Source: CAD feature listing. Evaluate the final solid. Frame: model axes, mm. A direction names the side the tool comes from. Give positions to 0.01 mm unless a question says otherwise; leave off trailing zeros. Write each loop counter-clockwise with the first axis right and the second up, starting at its lowest first coordinate (ties: lowest second). Pieces come first, ordered by that corner, then holes. Notation, with made-up numbers: (29.5, 30.25) -> (85.5, 30.25) arc R26 ccw to (85.5, 53.25) -> close; hole circle Ø11 at (57, 87.25). An arc over 180 degrees is marked (long way). Write item = value, one per line.
from build123d import *

# Parameters (mm, degrees)
SCHIZZO1_R                   = 3.4
ESTRUSIONE_ESTRUSIONE1_DEPTH = 200


with BuildPart() as part:
    # Schizzo1 → Estrusione-Estrusione1 (new body)
    with BuildSketch(Plane(origin=(0, 0, -1034), x_dir=(-1, 0, 0), z_dir=(0, 0, -1))):
        with BuildLine():
            Line((-16, 3.5), (-16, 1.5))
            ThreePointArc((-16, 1.5), (-15.560660172, 0.439339828), (-14.5, 0))
            Line((-14.5, 0), (-4, 0))
            ThreePointArc((-4, 0), (-1.171572875, 1.171572875), (0, 4))
            Line((0, 4), (0, 14.5))
            ThreePointArc((0, 14.5), (-0.439339828, 15.560660172), (-1.5, 16))
            Line((-1.5, 16), (-3.5, 16))
            ThreePointArc((-3.5, 16), (-4.207106781, 15.707106781), (-4.5, 15))
            Line((-4.5, 15), (-4.5, 13.5))
            ThreePointArc((-4.5, 13.5), (-4.353553391, 13.146446609), (-4, 13))
            Line((-4, 13), (-2.45, 13))
            ThreePointArc((-2.45, 13), (-2.131801948, 12.868198052), (-2, 12.55))
            Line((-2, 12.55), (-2, 12.5))
            ThreePointArc((-2, 12.5), (-2.732233047, 10.732233047), (-4.5, 10))
            Line((-4.5, 10), (-5.807611845, 10))
            ThreePointArc((-5.807611845, 10), (-7.721029007, 10.380602337), (-9.343145751, 11.464466094))
            Line((-9.343145751, 11.464466094), (-10.785533906, 12.906854249))
            ThreePointArc((-10.785533906, 12.906854249), (-11.869397663, 14.528970994), (-12.25, 16.442388155))
            Line((-12.25, 16.442388155), (-12.25, 23.557611845))
            ThreePointArc((-12.25, 23.557611845), (-11.869397663, 25.471029006), (-10.785533906, 27.09314575))
            Line((-10.785533906, 27.09314575), (-9.343145751, 28.535533906))
            ThreePointArc((-9.343145751, 28.535533906), (-7.721029006, 29.619397663), (-5.807611845, 30))
            Line((-5.807611845, 30), (-4.5, 30))
            ThreePointArc((-4.5, 30), (-2.732233047, 29.267766953), (-2, 27.5))
            Line((-2, 27.5), (-2, 27.45))
            ThreePointArc((-2, 27.45), (-2.131801948, 27.131801948), (-2.45, 27))
            Line((-2.45, 27), (-4, 27))
            ThreePointArc((-4, 27), (-4.353553391, 26.853553391), (-4.5, 26.5))
            Line((-4.5, 26.5), (-4.5, 25))
            ThreePointArc((-4.5, 25), (-4.207106781, 24.292893219), (-3.5, 24))
            Line((-3.5, 24), (-1.5, 24))
            ThreePointArc((-1.5, 24), (-0.439339828, 24.439339828), (0, 25.5))
            Line((0, 25.5), (0, 35.77708764))
            ThreePointArc((0, 35.77708764), (-1.333333333, 38.75851161), (-4.444444444, 39.7523196))
            ThreePointArc((-4.444444444, 39.7523196), (-28.284271247, 28.284271247), (-39.7523196, 4.444444444))
            ThreePointArc((-39.7523196, 4.444444444), (-38.75851161, 1.333333333), (-35.77708764, 0))
            Line((-35.77708764, 0), (-25.5, 0))
            ThreePointArc((-25.5, 0), (-24.439339828, 0.439339828), (-24, 1.5))
            Line((-24, 1.5), (-24, 3.5))
            ThreePointArc((-24, 3.5), (-24.292893219, 4.207106781), (-25, 4.5))
            Line((-25, 4.5), (-26.5, 4.5))
            ThreePointArc((-26.5, 4.5), (-26.853553391, 4.353553391), (-27, 4))
            Line((-27, 4), (-27, 2.45))
            ThreePointArc((-27, 2.45), (-27.131801948, 2.131801948), (-27.45, 2))
            Line((-27.45, 2), (-27.5, 2))
            ThreePointArc((-27.5, 2), (-29.267766953, 2.732233047), (-30, 4.5))
            Line((-30, 4.5), (-30, 5.807611845))
            ThreePointArc((-30, 5.807611845), (-29.619397663, 7.721029006), (-28.535533906, 9.343145751))
            Line((-28.535533906, 9.343145751), (-27.09314575, 10.785533906))
            ThreePointArc((-27.09314575, 10.785533906), (-25.471029006, 11.869397663), (-23.557611845, 12.25))
            Line((-23.557611845, 12.25), (-16.442388155, 12.25))
            ThreePointArc((-16.442388155, 12.25), (-14.528970994, 11.869397663), (-12.90685425, 10.785533906))
            Line((-12.90685425, 10.785533906), (-11.464466094, 9.343145751))
            ThreePointArc((-11.464466094, 9.343145751), (-10.380602337, 7.721029006), (-10, 5.807611845))
            Line((-10, 5.807611845), (-10, 4.5))
            ThreePointArc((-10, 4.5), (-10.732233047, 2.732233047), (-12.5, 2))
            Line((-12.5, 2), (-12.55, 2))
            ThreePointArc((-12.55, 2), (-12.868198052, 2.131801948), (-13, 2.45))
            Line((-13, 2.45), (-13, 4))
            ThreePointArc((-13, 4), (-13.146446609, 4.353553391), (-13.5, 4.5))
            Line((-13.5, 4.5), (-15, 4.5))
            ThreePointArc((-15, 4.5), (-15.707106781, 4.207106781), (-16, 3.5))
        make_face()
        with Locations(Location((-20, 20, 0), (0, 0, 180))):
            Circle(SCHIZZO1_R, mode=Mode.SUBTRACT)
        with BuildLine():
            Line((-8.2, 32.3), (-8.2, 36.905284174))
            ThreePointArc((-8.2, 36.905284174), (-8.087982608, 37.220672025), (-7.802122016, 37.394744177))
            ThreePointArc((-7.802122016, 37.394744177), (-6.029991855, 37.721071011), (-4.244444444, 37.963465218))
            ThreePointArc((-4.244444444, 37.963465218), (-2.533333333, 37.416870823), (-1.8, 35.77708764))
            Line((-1.8, 35.77708764), (-1.8, 32.3))
            ThreePointArc((-1.8, 32.3), (-1.946446609, 31.946446609), (-2.3, 31.8))
            Line((-2.3, 31.8), (-7.7, 31.8))
            ThreePointArc((-7.7, 31.8), (-8.053553391, 31.946446609), (-8.2, 32.3))
        make_face(mode=Mode.SUBTRACT)
        with BuildLine():
            Line((-4, 1.8), (-7.7, 1.8))
            ThreePointArc((-7.7, 1.8), (-8.053553391, 1.946446609), (-8.2, 2.3))
            Line((-8.2, 2.3), (-8.2, 7.7))
            ThreePointArc((-8.2, 7.7), (-8.053553391, 8.053553391), (-7.7, 8.2))
            Line((-7.7, 8.2), (-2.3, 8.2))
            ThreePointArc((-2.3, 8.2), (-1.946446609, 8.053553391), (-1.8, 7.7))
            Line((-1.8, 7.7), (-1.8, 4))
            ThreePointArc((-1.8, 4), (-2.444365081, 2.444365081), (-4, 1.8))
        make_face(mode=Mode.SUBTRACT)
        with BuildLine():
            Line((-27.75, 23.606725737), (-27.75, 16.442388155))
            ThreePointArc((-27.75, 16.442388155), (-28.130602337, 14.528970994), (-29.214466094, 12.906854249))
            Line((-29.214466094, 12.906854249), (-30.656854249, 11.464466094))
            ThreePointArc((-30.656854249, 11.464466094), (-32.278970994, 10.380602337), (-34.192388155, 10))
            Line((-34.192388155, 10), (-36.208286344, 10))
            ThreePointArc((-36.208286344, 10), (-36.608054182, 10.199690699), (-36.688502344, 10.639257294))
            ThreePointArc((-36.688502344, 10.639257294), (-33.797037909, 17.804500235), (-29.522849462, 24.241315138))
            ThreePointArc((-29.522849462, 24.241315138), (-28.412990699, 24.548227054), (-27.75, 23.606725737))
        make_face(mode=Mode.SUBTRACT)
        with BuildLine():
            Line((-10, 36.208286344), (-10, 34.192388155))
            ThreePointArc((-10, 34.192388155), (-10.380602337, 32.278970994), (-11.464466094, 30.656854249))
            Line((-11.464466094, 30.656854249), (-12.906854249, 29.214466094))
            ThreePointArc((-12.906854249, 29.214466094), (-14.528970994, 28.130602337), (-16.442388155, 27.75))
            Line((-16.442388155, 27.75), (-23.606725737, 27.75))
            ThreePointArc((-23.606725737, 27.75), (-24.548227054, 28.412990699), (-24.241315138, 29.522849462))
            ThreePointArc((-24.241315138, 29.522849462), (-17.804500235, 33.797037909), (-10.639257294, 36.688502344))
            ThreePointArc((-10.639257294, 36.688502344), (-10.199690699, 36.608054182), (-10, 36.208286344))
        make_face(mode=Mode.SUBTRACT)
        with BuildLine():
            Line((-36.905284174, 8.2), (-32.3, 8.2))
            ThreePointArc((-32.3, 8.2), (-31.946446609, 8.053553391), (-31.8, 7.7))
            Line((-31.8, 7.7), (-31.8, 2.3))
            ThreePointArc((-31.8, 2.3), (-31.946446609, 1.946446609), (-32.3, 1.8))
            Line((-32.3, 1.8), (-35.77708764, 1.8))
            ThreePointArc((-35.77708764, 1.8), (-37.416870823, 2.533333333), (-37.963465218, 4.244444444))
            ThreePointArc((-37.963465218, 4.244444444), (-37.721071011, 6.029991855), (-37.394744177, 7.802122016))
            ThreePointArc((-37.394744177, 7.802122016), (-37.220672025, 8.087982608), (-36.905284174, 8.2))
        make_face(mode=Mode.SUBTRACT)
    extrude(amount=-ESTRUSIONE_ESTRUSIONE1_DEPTH)


solid = part.part
1) Cut plane C-C (z = -853.5). State how many separate pieces and enclosed holes the cut face has, then the cut area to 3 significant figures.
Computed:
separate_pieces = 1
enclosed_holes = 6
area = 575 mm²
2) Draft query along X for faces 3 (the cylindrical face through (38.79, 1.37, -935.4)), 4 (the cylindrical face through (19.26, 23.32, -935.4)), 5 (the flat face through (16, 17, -834)), 6 (the cylindrical face through (32.254, 10.391, -935.4)). Return one class per face: pulls with the +X half, pulls with the -X half, needs draft (parallel to the pull), parting line crosses it, or undercut.
Computed:
face_3 = pulls with the +X half
face_4 = undercut
face_5 = needs draft
face_6 = undercut
3) Access query for faces 1 (the flat face through (0, 31, -935)), 2 (the flat face through (5, 31.8, -935)). Directions: +Z, -Z, +X, -X, +Y, -Y. A direction counts if a zero-diameter tool reaches every point of the face in a straight line with its end or side. Return the directions, or none.
Computed:
face_1 = +Z, -Z, -X, +Y, -Y
face_2 = +Z, -Z
4) Contact query for flat-ended pins moving along their axis: pin 1 (3 mm diameter, centred on y = 34.5, z = -947, fed in from +X); pin 2 (4 mm diameter, centred on y = 10, z = -1004.5, fed in from +X); pin 3 (0.6 mm diameter, centred on x = 35, z = -981, fed in from +Y). Output: stop coordinate, or through.
Computed:
pin_1 = 22.61
pin_2 = 39.19
pin_3 = 19.9
5) Cut plane A-A (y = 20). Return the cut outline in (x, z), then the cut area to 3 significant figures.
Computed:
outline = (12.25, -1034) -> (16.6, -1034) -> (16.6, -834) -> (12.25, -834) -> close; (23.4, -1034) -> (27.75, -1034) -> (27.75, -834) -> (23.4, -834) -> close; (32.55, -1034) -> (34.64, -1034) -> (34.64, -834) -> (32.55, -834) -> close
area = 2,160 mm²
6) Material intervals for L1, parallel to Y at x = 6, z = -1000; L2, parallel to X at y = 28.5, z = -1001; L3, parallel to X at y = 20, z = -927, sorted ascending.
Computed:
L1 = 0 to 1.8, 8.2 to 10, 30 to 31.8, 37.73 to 39.55
L2 = 0 to 2.21, 9.38 to 13.81, 24.57 to 28.07
L3 = 12.25 to 16.6, 23.4 to 27.75, 32.55 to 34.64
